Input: part model. Units: mm. Frame: model coordinates. Face numbers are marked on the shaded views. A direction names the side the tool comes from. Coordinates: 2 decimals unless noted, no trailing zeros. Write each loop counter-clockwise with the first axis right and the second up, starting at its lowest first coordinate (ties: lowest second). Pieces come first, ordered by that corner, then holes. Notation, with made-up numbers: (15, -20) - (20, -20) arc R15 cw to (20, 5) - close; hole circle Ø5 at (23, 38.5). An arc over 180 degrees is marked (long way). Use a Markdown table: item, result. Add a question column.
Q1. Material intervals for probe 1 along Y at (x, z) = (0, 100.8); probe 2 along Z at (x, y) = (8, 1); probe 3 along Z at (x, y) = (1.25, 0), sorted ascending. Write a range as from..to.
Q2. Section query B-B (z = 15). Return the cut outline in (x, y).
Q3. Pin query (flat end, axial travel): P1, Ø5, axis at x = -3, z = 90, coming from the +Y side; P2, Ø5, axis at x = -6.5, z = 41, coming from the +Y side; P3, Ø1.4, axis at x = 6, z = 32, coming from the -Y side. Return the tip coordinate at first contact, or that it passes through.
Q4. Section query A-A (x = 0). Return the cut outline in (y, z), then the cut area to 3 significant figures.
Q5. Set-up query: the marked faces 1, 2 and 3. Return all of +Z, -Z, +X, -X, +Y, -Y with unobstructed straight access to the full face (end or side cutting, diameter ignored); none if empty.
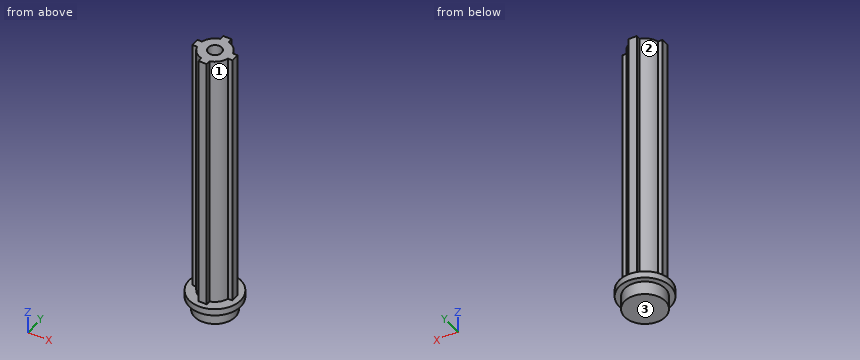
from build123d import *

# Parameters (mm, degrees)
SKETCH1_R           = 7.5
BOSS_EXTRUDE1_DEPTH = 5
SKETCH3_R           = 9.5
BOSS_EXTRUDE2_DEPTH = 2.5
BOSS_EXTRUDE3_DEPTH = 96
SKETCH5_R           = 2.5
CUT_EXTRUDE1_DEPTH  = 5


with BuildPart() as part:
    # Sketch1 → Boss-Extrude1 (new body)
    with BuildSketch(Plane.XY):
        Circle(SKETCH1_R)
    extrude(amount=BOSS_EXTRUDE1_DEPTH)

    # Sketch3 → Boss-Extrude2 (add)
    with BuildSketch(Plane.XY.offset(5)):
        Circle(SKETCH3_R)
    extrude(amount=BOSS_EXTRUDE2_DEPTH)

    # Sketch4 → Boss-Extrude3 (add)
    with BuildSketch(Plane.XY.offset(7.5)):
        with BuildLine():
            Line((-1.5, 5.652839314), (-1.5, 7.348469228))
            Line((-1.5, 7.348469228), (1.5, 7.348469228))
            Line((1.5, 7.348469228), (1.5, 5.652839314))
            ThreePointArc((1.5, 5.652839314), (4.135492251, 4.135492251), (5.652839314, 1.5))
            Line((5.652839314, 1.5), (7.348469228, 1.5))
            Line((7.348469228, 1.5), (7.348469228, -1.5))
            Line((7.348469228, -1.5), (5.652839314, -1.5))
            ThreePointArc((5.652839314, -1.5), (4.135492251, -4.135492251), (1.5, -5.652839314))
            Line((1.5, -5.652839314), (1.5, -7.348469228))
            Line((1.5, -7.348469228), (-1.5, -7.348469228))
            Line((-1.5, -7.348469228), (-1.5, -5.652839314))
            ThreePointArc((-1.5, -5.652839314), (-4.135492251, -4.135492251), (-5.652839314, -1.5))
            Line((-5.652839314, -1.5), (-7.348469228, -1.5))
            Line((-7.348469228, -1.5), (-7.348469228, 1.5))
            Line((-7.348469228, 1.5), (-5.652839314, 1.5))
            ThreePointArc((-5.652839314, 1.5), (-4.135492251, 4.135492251), (-1.5, 5.652839314))
        make_face()
    extrude(amount=BOSS_EXTRUDE3_DEPTH)

    # Sketch5 → Cut-Extrude1 (cut)
    with BuildSketch(Plane.XY.offset(103.5)):
        Circle(SKETCH5_R)
    extrude(amount=-CUT_EXTRUDE1_DEPTH, mode=Mode.SUBTRACT)


solid = part.part
Values follow:
| question | item | result |
|---|---|---|
| 1 | probe 1 | -7.35..-2.5, 2.5..7.35 |
| 1 | probe 2 | 5..7.5 |
| 1 | probe 3 | 0..98.5 |
| 2 | outline | (-7.35, -1.5) - (-5.65, -1.5) arc R5.85 ccw to (-1.5, -5.65) - (-1.5, -7.35) - (1.5, -7.35) - (1.5, -5.65) arc R5.85 ccw to (5.65, -1.5) - (7.35, -1.5) - (7.35, 1.5) - (5.65, 1.5) arc R5.85 ccw to (1.5, 5.65) - (1.5, 7.35) - (-1.5, 7.35) - (-1.5, 5.65) arc R5.85 ccw to (-5.65, 1.5) - (-7.35, 1.5) - close |
| 3 | P1 | y = 7.35 |
| 3 | P2 | y = 4.27 |
| 3 | P3 | y = -2.47 |
| 4 | outline | (-9.5, 5) - (-7.5, 5) - (-7.5, 0) - (7.5, 0) - (7.5, 5) - (9.5, 5) - (9.5, 7.5) - (7.35, 7.5) - (7.35, 103.5) - (2.5, 103.5) - (2.5, 98.5) - (-2.5, 98.5) - (-2.5, 103.5) - (-7.35, 103.5) - (-7.35, 7.5) - (-9.5, 7.5) - close |
| 4 | area | 1,510 mm2 |
| 5 | face 1 | +Z, +X, -Y |
| 5 | face 2 | +Z, -X, +Y |
| 5 | face 3 | -Z, +X, -X, +Y, -Y |
